Solid Edge part; units mm, degrees
sketch "Sketch1" plane through (0, 0, 0) normal (0, -1, 0) x (1, 0, 0)
  line L0 (0, 15) -> (0, -15)
  line L1 (0, -15) -> (30, -15)
  line L2 (30, -15) -> (30, -13)
  line L3 (30, -13) -> (2, -13)
  line L4 (2, -13) -> (2, 13)
  line L5 (2, 13) -> (30, 13)
  line L6 (30, 13) -> (30, 15)
  line L7 (30, 15) -> (0, 15)
  dimension "D1" = 30
  dimension "D2" = 30
extrude "Protrusion1" add sketch "Sketch1" along normal mid plane 100
properties material "Aluminum, 1060"
Design review of the part built by this model. Coordinates are the model's own, in mm. A direction names the side the tool comes from. Give positions to 0.01 mm unless a question says otherwise; leave off trailing zeros. Loops run counter-clockwise (first coordinate to the right, second up) from the corner with the lowest first, then second, coordinate; pieces in that order, holes last. Notation, with made-up numbers: (21, 80.5) - (41, 80.5) arc R22 ccw to (41, 106.5) - close; hole circle Ø8 at (49, -8). An arc over 180 degrees is marked (long way). Write item = value, one per line.
1) To check wall thickness, follow line 1 (Z direction, x = 21.75, y = 14); line 2 (X direction, y = -33, z = 10.25). State the ranges of each line that lie inside material, in increasing order.
Result sheet:
line_1 = -15 to -13, 13 to 15
line_2 = 0 to 2
2) Take a section at A-A on x = 27. State the section outline as (y, z) points, and give its area (3 significant figures).
Result sheet:
outline = (-50, -15) - (50, -15) - (50, -13) - (-50, -13) - close; (-50, 13) - (50, 13) - (50, 15) - (-50, 15) - close
area = 400 mm2
3) Take a section at B-B on y = -30. State the section outline as (x, z) points.
Result sheet:
outline = (0, -15) - (30, -15) - (30, -13) - (2, -13) - (2, 13) - (30, 13) - (30, 15) - (0, 15) - close
4) Draft analysis for pull direction Z (two halves, no side actions). For faces 1 (the face through (15, 1, -15)), 2 (the face through (0, 1, 0)), 3 (the face through (16, 1, -13)), state which applies: +Z half, -Z half, draft (parallel to the pull), parting line (faces both ways), or undercut.
Result sheet:
face_1 = -Z half
face_2 = draft
face_3 = undercut
5) Take a section at C-C on z = 6. State the section outline as (x, y) points.
Result sheet:
outline = (0, -50) - (2, -50) - (2, 50) - (0, 50) - close
6) Clearance check with a flat-ended pin moving along its axis: pin 1 Ø10 at (y, z) = (-5, -0.5) entering from +X. State where the tip first meets the part, or that it passes through.
Result sheet:
pin_1 = 2
7) Tool access review of faces 4 (the face through (16, 1, 13)), 5 (the face through (30, 1, 14)): name each direction out of +Z, -Z, +X, -X, +Y, -Y from which nothing blocks a thin tool from reaching the whole face with its end or side.
Result sheet:
face_4 = +X, +Y, -Y
face_5 = +Z, -Z, +X, +Y, -Y
